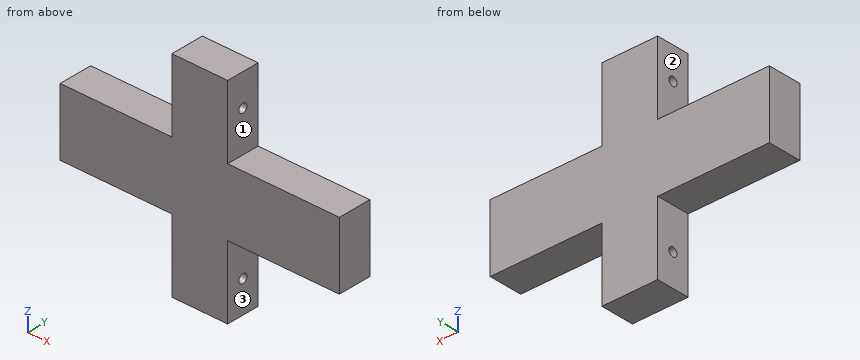
```python
from build123d import *

# Parameters (mm, degrees)
BOSS_EXTRUDE1_DEPTH     = 60
CUT_EXTRUDE1_DEPTH      = 361.138862107
CUT_EXTRUDE1_DEPTH_BACK = 361.138862107
SKETCH2_R               = 8


with BuildPart() as part:
    # Sketch1 → Boss-Extrude1 (new body)
    with BuildSketch(Plane(origin=(0, 0, 0), x_dir=(1, 0, 0), z_dir=(0, 1, 0))):
        Polygon((-250, 60), (-50, 60), (-50, 190), (50, 190), (50, 60), (250, 60), (250, -60), (50, -60), (50, -190), (-50, -190), (-50, -60), (-250, -60), align=None)
    extrude(amount=BOSS_EXTRUDE1_DEPTH)

    # Sketch2 → Cut-Extrude1 (cut, two sides: drawn at the far end of the back side and taken through both)
    with BuildSketch(Plane.ZY.offset(50).offset(-CUT_EXTRUDE1_DEPTH_BACK)):
        with Locations((133, 30)):
            Circle(SKETCH2_R)
        with Locations((-133, 30)):
            Circle(SKETCH2_R)
    extrude(amount=CUT_EXTRUDE1_DEPTH + CUT_EXTRUDE1_DEPTH_BACK, mode=Mode.SUBTRACT)


solid = part.part
```
For this review, take the finished solid that the model builds, in its own axes (mm). Face numbers are marked on the shaded views. A direction names the side the tool comes from. Give positions to 0.01 mm unless a question says otherwise; leave off trailing zeros. Write each loop counter-clockwise with the first axis right and the second up, starting at its lowest first coordinate (ties: lowest second). Pieces come first, ordered by that corner, then holes. Notation, with made-up numbers: M 26,28.5 L 41,28.5 A13 cw 41,45.5 Z; hole C 75.5,-12.5 d1. An arc over 180 degrees is marked long. One line per item, written item: value.
1) For line 1 (Z direction, x = 19.5, y = 30); line 2 (Y direction, x = -9, z = 133); line 3 (Z direction, x = 42.5, y = 26), list the stretches that pass through material, from the lowest coordinate up. Write a range as from..to.
Results are:
line 1: z = -190..-141, -125..125, 141..190
line 2: y = 0..22, 38..60
line 3: z = -190..-139.93, -126.07..126.07, 139.93..190
2) Take a section at C-C, the plane x = -21. Write out the cut boundary in (y, z).
Results are:
outline: M 0,-190 L 60,-190 L 60,190 L 0,190 Z; hole C 30,-133 d16; hole C 30,133 d16
3) Take a section at D-D, the plane x = -186.5. Write out the cut boundary in (y, z), then the cut area to 3 significant figures.
Results are:
outline: M 0,-60 L 60,-60 L 60,60 L 0,60 Z
area: 7,200 mm²
4) Take a section at A-A, the plane z = -133. Write out the cut boundary in (x, y), then the cut area to 3 significant figures.
Results are:
outline: M -50,0 L 50,0 L 50,22 L -50,22 Z; M -50,38 L 50,38 L 50,60 L -50,60 Z
area: 4,400 mm²
5) For P1, Ø9.5, axis at y = 30, z = 133, coming from the +X side; P2, Ø12, axis at x = -132.5, y = 38.5, coming from the +Z side; P3, Ø18.5, axis at y = 30, z = -133, coming from the -X side; P4, Ø18, axis at y = 42, z = -135, coming from the +X side, all flat-tipped, find the tip position at first contact; note any pin that passes through.
Results are:
P1: passes through
P2: stops at z = 60
P3: stops at x = -50
P4: stops at x = 50
6) For the marked faces 1, 2 and 3, list the 3-axis set-ups (+Z, -Z, +X, -X, +Y, -Y) from which the entire face can be reached by the end or side of a thin tool; tool diameter is ignored.
Results are:
face 1: +Z, +X, +Y, -Y
face 2: +Z, -X, +Y, -Y
face 3: -Z, +X, +Y, -Y
7) Take a section at B-B, the plane y = 9.5. Write out the cut boundary in (x, z), then the cut area to 3 significant figures.
Results are:
outline: M -250,-60 L -50,-60 L -50,-190 L 50,-190 L 50,-60 L 250,-60 L 250,60 L 50,60 L 50,190 L -50,190 L -50,60 L -250,60 Z
area: 86,000 mm²
